For this review, use the dimensioned drawing (mm, ordinates from the lowest corner) and the shaded views. Round coordinates to 2 decimals unless told otherwise and drop trailing zeros. Write each loop counter-clockwise with the first axis right and the second up, starting at its lowest first coordinate (ties: lowest second). Pieces come first, ordered by that corner, then holes. Notation, with made-up numbers: (52.25, 3.25) -> (100.25, 3.25) arc R24 ccw to (100.25, 31.25) -> close; hole circle Ø9 at (10.5, 42). An arc over 180 degrees is marked (long way). Answer as CSV lines item,"result". Start each with the question number.
Item 1: Take a section at A-A on x = 7.5. Give the boundary of the cut face in (y, z).
Item 2: Wall thickness on probe 1 along Z at (x, y) = (7.5, 3.8); probe 2 along X at (y, z) = (3.85, 10); probe 3 along Z at (x, y) = (33.5, 2.5): over which ranges is each line inside the solid? List them lowest first. Write a range as from..to.
Item 3: For pin 1 Ø5 at (x, z) = (7.5, 10) entering from -Y; pin 2 Ø6.5 at (x, z) = (7.5, 40) entering from +Y, all flat-tipped, find the tip position at first contact; note any pin that passes through.
Item 4: Take a section at D-D on z = 40. Give the boundary of the cut face in (x, y).
Item 5: Take a section at B-B on z = 25. Give the boundary of the cut face in (x, y).
Item 6: Mouldability with a two-part tool opening along X and no side actions: class the marked faces 1, 2 and 3 as +X half, -X half, draft (parallel to the pull), parting line (faces both ways), or undercut.
Item 7: Take a section at C-C on x = 20. Give the boundary of the cut face in (y, z), then the cut area to 3 significant figures.
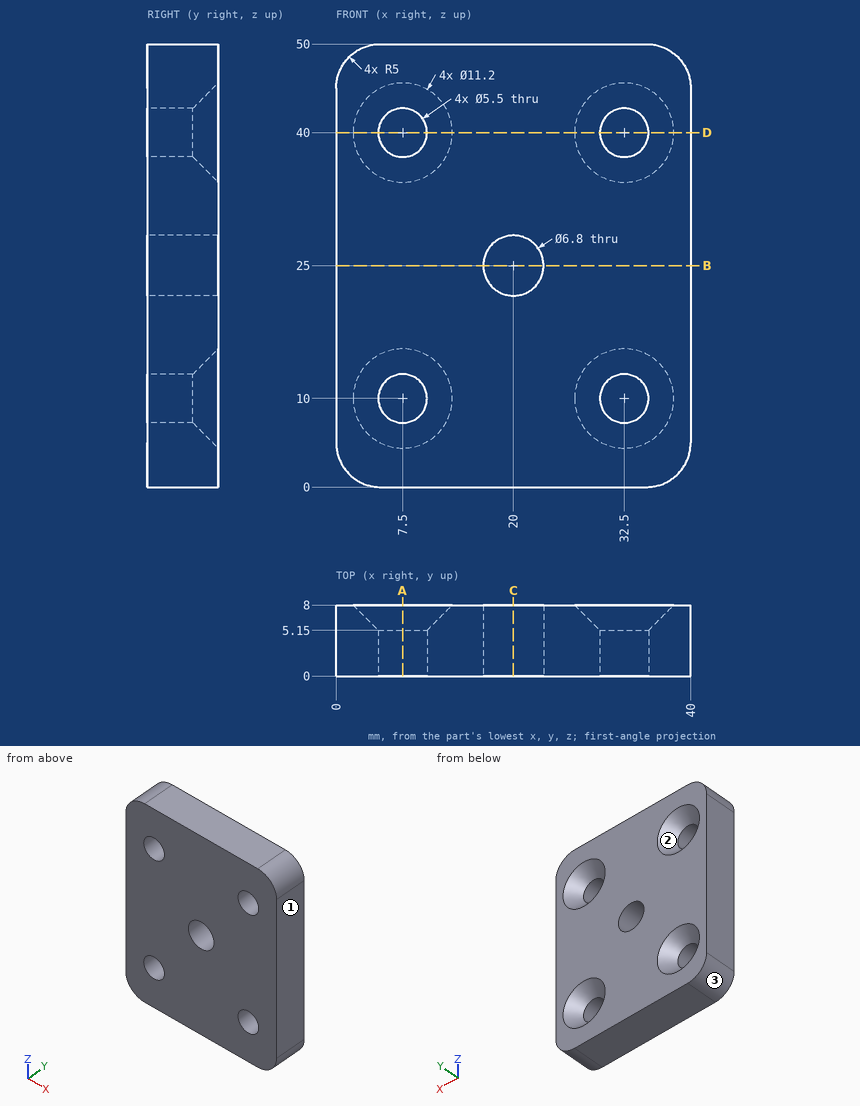
Output values:
1,outline,"(0, 0) -> (8, 0) -> (8, 4.4) -> (5.15, 7.25) -> (0, 7.25) -> close; (0, 12.75) -> (5.15, 12.75) -> (8, 15.6) -> (8, 34.4) -> (5.15, 37.25) -> (0, 37.25) -> close; (0, 42.75) -> (5.15, 42.75) -> (8, 45.6) -> (8, 50) -> (0, 50) -> close"
2,probe 1,"z = 0..7.25, 12.75..37.25, 42.75..50"
2,probe 2,"x = 0..4.75, 10.25..29.75, 35.25..40"
2,probe 3,"z = 0..7.44, 12.56..37.44, 42.56..50"
3,pin 1,"passes through"
3,pin 2,"stops at y = 5.65"
4,outline,"(0, 0) -> (4.75, 0) -> (4.75, 5.15) -> (1.9, 8) -> (0, 8) -> close; (10.25, 0) -> (29.75, 0) -> (29.75, 5.15) -> (26.9, 8) -> (13.1, 8) -> (10.25, 5.15) -> close; (35.25, 0) -> (40, 0) -> (40, 8) -> (38.1, 8) -> (35.25, 5.15) -> close"
5,outline,"(0, 0) -> (16.6, 0) -> (16.6, 8) -> (0, 8) -> close; (23.4, 0) -> (40, 0) -> (40, 8) -> (23.4, 8) -> close"
6,face 1,"+X half"
6,face 2,"undercut"
6,face 3,"-X half"
7,outline,"(0, 0) -> (8, 0) -> (8, 21.6) -> (0, 21.6) -> close; (0, 28.4) -> (8, 28.4) -> (8, 50) -> (0, 50) -> close"
7,area,"346 mm^2"
